from build123d import *

# Parameters (mm, degrees)
BOSS_EXTRUDE1_DEPTH = 1.5
BOSS_EXTRUDE2_DEPTH = 2
FILLET1_R           = 1
FILLET2_R           = 1
SKETCH3_R           = 3.25
CUT_EXTRUDE1_DEPTH  = 4.5
SKETCH4_R           = 0.75
CUT_EXTRUDE2_DEPTH  = 2.5


with BuildPart() as part:
    # Sketch1 → Boss-Extrude1 (new body)
    with BuildSketch(Plane(origin=(0, 0, 0), x_dir=(1, 0, 0), z_dir=(0, 1, 0))):
        Polygon((-10.65, 18), (-4, 11), (-4, 0), (4, 0), (4, 11), (10.65, 18), (10.65, 24.5), (-10.65, 24.5), align=None)
    extrude(amount=BOSS_EXTRUDE1_DEPTH)

    # Sketch2 → Boss-Extrude2 (add)
    with BuildSketch(Plane.XZ):
        with BuildLine():
            Line((4, 0), (4, -12.5))
            ThreePointArc((4, -12.5), (0, -20.5), (-4, -12.5))
            Line((-4, -12.5), (-4, 0))
            Line((-4, 0), (4, 0))
        make_face()
    extrude(amount=BOSS_EXTRUDE2_DEPTH)

    # Fillet1
    fillet1_edges = [part.edges().sort_by_distance(p)[0] for p in [
        (0, -2, 0),
        (-4, -2, -6.25),
        (0, -2, -20.5),
        (4, -2, -6.25),
    ]]
    fillet(fillet1_edges, radius=FILLET1_R)

    # Fillet2
    fillet2_edges = [part.edges().sort_by_distance(p)[0] for p in [
        (-7.325, 0, -14.5),
        (-10.65, 0, -21.25),
        (10.65, 0, -21.25),
        (7.325, 0, -14.5),
    ]]
    fillet(fillet2_edges, radius=FILLET2_R)

    # Sketch3 → Cut-Extrude1 (cut, through all)
    with BuildSketch(Plane.XZ.offset(2)):
        with Locations((0, -15.5)):
            Circle(SKETCH3_R)
    extrude(amount=-CUT_EXTRUDE1_DEPTH, mode=Mode.SUBTRACT)

    # Sketch4 → Cut-Extrude2 (cut, through all)
    with BuildSketch(Plane.XZ):
        with Locations((-8.5, -21.5)):
            Circle(SKETCH4_R)
        with Locations((8.5, -21.5)):
            Circle(SKETCH4_R)
    extrude(amount=-CUT_EXTRUDE2_DEPTH, mode=Mode.SUBTRACT)


solid = part.part
Build history of the part. All positions in model axes, mm. A direction names the side the tool comes from. Give positions to 0.01 mm unless a question says otherwise; leave off trailing zeros. Write each loop counter-clockwise with the first axis right and the second up, starting at its lowest first coordinate (ties: lowest second). Pieces come first, ordered by that corner, then holes. Notation, with made-up numbers: (66.5, 40) - (95.5, 40) arc R7 ccw to (95.5, 48) - close; hole circle Ø11 at (-3, 29.5). An arc over 180 degrees is marked (long way). Use one line per item in the form item = value. Start each with the question number.
1. Drop a flat-ended pin along its axis: pin 1 Ø0.8 at (y, z) = (-0.5, -7.5) entering from -X. Give the stop position or say it passes through.
2. 3-axis set-ups, long thin cutter, end or side, ignore diameter. For faces 1 (the face through (-3.715, -1.699, -6.337)), 2 (the face through (0.155, -0.493, -20.498)), 3 (the face through (0, -2, -8)), 4 (the face through (3.715, -1.699, -6.517)), 5 (the face through (-0.423, -0.274, -12.278)): which of +Z, -Z, +X, -X, +Y, -Y reach the whole face in a straight line?
3. Two-plate mould, pull along X, no slides. Class faces 6 (the face through (10.349, 0.285, -21.296)), 7 (the face through (-8.663, 0.74, -22.232)), 8 (the face through (0, 0, 0)): released by +X, released by -X, zero draft, split by the parting line, or undercut.
4. Band-saw the part on C-C on z = -6.75. Write the cut outline in (x, y).
5. Band-saw the part on B-B on x = 0. Write the cut outline in (y, z).
6. Band-saw the part on A-A on z = -21.5. Write the cut outline in (x, y), plus the area to 3 significant figures.
7. Probe line 1 (Y direction, x = 8.5, z = -22.5); line 2 (X direction, y = -0.9, z = -3); line 3 (Z direction, x = 8.5, y = 0.5). List the from-to ranges inside material, lowest first. Write a range as [from, to].
Conclusion:
q1.pin_1 = -4
q2.face_1 = +Z, -X, -Y
q2.face_2 = -Y
q2.face_3 = +Z, -Z, +X, -X, -Y
q2.face_4 = +Z, +X, -Y
q2.face_5 = +Y, -Y
q3.face_6 = released by +X
q3.face_7 = undercut
q3.face_8 = zero draft
q4.outline = (-4, -1) arc R1 ccw to (-3, -2) - (3, -2) arc R1 ccw to (4, -1) - (4, 1.5) - (-4, 1.5) - close
q5.outline = (-2, -19.5) arc R1 ccw to (-1, -20.5) - (0, -20.5) - (0, -24.5) - (1.5, -24.5) - (1.5, -18.75) - (-2, -18.75) - close; (-2, -12.25) - (1.5, -12.25) - (1.5, 0) - (-1, 0) arc R1 ccw to (-2, -1) - close
q6.outline = (-10.65, 1) arc R1 ccw to (-9.65, 0) - (-9.25, 0) - (-9.25, 1.5) - (-10.65, 1.5) - close; (-7.75, 0) - (7.75, 0) - (7.75, 1.5) - (-7.75, 1.5) - close; (9.25, 0) - (9.65, 0) arc R1 ccw to (10.65, 1) - (10.65, 1.5) - (9.25, 1.5) - close
q6.area = 27.0 mm²
q7.line_1 = [0, 1.5]
q7.line_2 = [-4, 4]
q7.line_3 = [-24.5, -22.25], [-20.75, -15.93]
